Design review of the part built by this model. Coordinates are the model's own, in mm. A direction names the side the tool comes from. Round coordinates to 2 decimals unless told otherwise and drop trailing zeros. Loops run counter-clockwise (first coordinate to the right, second up) from the corner with the lowest first, then second, coordinate; pieces in that order, holes last. Notation, with made-up numbers: (6.25, 88.5) -> (25.25, 88.5) arc R29 ccw to (25.25, 117.5) -> close; hole circle Ø2 at (-39, -1). An arc over 180 degrees is marked (long way). Answer as CSV lines item,"result". Start each with the question number.
(1) Machinability: for faces 4 (the face through (-1.734, 2.262, 145.653)), 5 (the face through (-2.737, 1.61, 72.666)), 6 (the face through (0, -3.175, 73)), 7 (the face through (2.737, -1.61, 72.666)), which of the approach directions +Z, -Z, +X, -X, +Y, -Y give a long, thin tool a straight path to every point of the face, cutting with its end or side? Answer none if there is none.
(2) Take a section at C-C, the plane y = 4.5. Write out the cut boundary in (x, z), and give its area (3 significant figures).
(3) To check wall thickness, follow line 1 (Z direction, x = -6, y = -4); line 2 (Y direction, x = -3.5, z = 48); line 3 (X direction, y = 0.5, z = 144.5). State the ranges of each line that lie inside material, in increasing order. Write a range as from..to.
(4) Draft analysis for pull direction Z (two halves, no side actions). For faces 1 (the face through (0, 0, 159.012)), 2 (the face through (-2.76, -1.57, 72.67)), 3 (the face through (0, 3, 146.312)), state which applies: +Z half, -Z half, draft (parallel to the pull), parting line (faces both ways), or undercut.
(5) Take a section at A-A, the plane x = 0. Write out the cut boundary in (y, z) (3 decimals), and give its area (3 significant figures).
(6) Take a section at B-B, the plane z = 76. Write out the cut boundary in (x, y) (3 decimals).
(7) For P1, Ø4, axis at x = -2.5, z = 112.5, coming from the +Y side (3 decimals); P2, Ø2, axis at x = 1.5, z = 57, coming from the -Y side (3 decimals); P3, Ø6, axis at y = 3.5, z = 107.5, coming from the -X side, all flat-tipped, find the tip position at first contact; note any pin that passes through.
from build123d import *

# Parameters (mm, degrees)
SKETCH1_R          = 9.35
PISTON_DEPTH       = 2.5
ROD_DEPTH          = 159.0119
SKETCH4_R          = 9.35
SKETCH4_R_2        = 3.175
THREAD_DEPTH       = 14
CHAMFER1_SIZE      = 1
SKETCH5_W          = 1.3
SKETCH5_H          = 2.54
CUT_REVOLVE1_ANGLE = 180


with BuildPart() as part:
    # Sketch1 → Piston (new, symmetric)
    with BuildSketch(Plane.XY):
        Circle(SKETCH1_R)
    extrude(amount=PISTON_DEPTH, both=True)

    # Sketch2 → Rod (add)
    with BuildSketch(Plane.XY):
        Polygon((3.666174209, 0), (1.833087105, 3.175), (-1.833087105, 3.175), (-3.666174209, 0), (-1.833087105, -3.175), (1.833087105, -3.175), align=None)
    extrude(amount=ROD_DEPTH)

    # Sketch4 → Thread (cut)
    with BuildSketch(Plane.XY.offset(159.0119)):
        Circle(SKETCH4_R)
        with Locations(Location((0, 0, 0), (0, 0, 330))):
            Circle(SKETCH4_R_2, mode=Mode.SUBTRACT)
    extrude(amount=-THREAD_DEPTH, mode=Mode.SUBTRACT)

    # Chamfer1
    chamfer1_edges = [part.edges().sort_by_distance(p)[0] for p in [
        (-2.749630657, 1.5875, 159.0119),
    ]]
    chamfer(chamfer1_edges, length=CHAMFER1_SIZE)

    # Sketch5 → Cut-Revolve1 (revolve, cut)
    with BuildSketch(Plane(origin=(0, 0, 0), x_dir=(0, 0, -1), z_dir=(1, 0, 0))):
        with Locations((-145.6619, 4.12)):
            Rectangle(SKETCH5_W, SKETCH5_H)
        with Locations((-145.6619, -4.12)):
            Rectangle(SKETCH5_W, SKETCH5_H)
    revolve(axis=Axis((0, 0, 47.288533753), (0, 0, 1)), revolution_arc=CUT_REVOLVE1_ANGLE, mode=Mode.SUBTRACT)

    # Sketch6 → Cut-Revolve2 (revolve, cut)
    with BuildSketch(Plane(origin=(0, 0, 0), x_dir=(0, 0, -1), z_dir=(1, 0, 0)), mode=Mode.PRIVATE) as cut_revolve2_sk:
        Polygon((-145.0119, 2.85), (-145.0119, 7.746831352), (-142.184713101, 7.746831352), align=None)
    revolve(cut_revolve2_sk.sketch.rotate(Axis((0, 0, 96.043182271), (0, 0, 1)), 90), axis=Axis((0, 0, 96.043182271), (0, 0, 1)), mode=Mode.SUBTRACT)


solid = part.part
The answers:
1,face 4,"none"
1,face 5,"+Z, -X, +Y"
1,face 6,"+Z, +X, -X, -Y"
1,face 7,"+Z, +X, -Y"
2,outline,"(-8.2, -2.5) -> (8.2, -2.5) -> (8.2, 2.5) -> (-8.2, 2.5) -> close"
2,area,"82.0 mm²"
3,line 1,"-2.5..2.5"
3,line 2,"-0.29..0.29"
3,line 3,"-3.38..3.38"
4,face 1,"+Z half"
4,face 2,"draft"
4,face 3,"undercut"
5,outline,"(-9.35, -2.5) -> (9.35, -2.5) -> (9.35, 2.5) -> (3.175, 2.5) -> (3.175, 144.824) -> (2.85, 145.012) -> (2.85, 146.312) -> (3.175, 146.312) -> (3.175, 158.012) -> (2.175, 159.012) -> (-2.175, 159.012) -> (-3.175, 158.012) -> (-3.175, 146.312) -> (-2.85, 146.312) -> (-2.85, 145.012) -> (-3.175, 144.824) -> (-3.175, 2.5) -> (-9.35, 2.5) -> close"
5,area,"1,090 mm²"
6,outline,"(-3.666, 0) -> (-1.833, -3.175) -> (1.833, -3.175) -> (3.666, 0) -> (1.833, 3.175) -> (-1.833, 3.175) -> close"
7,P1,"y = 3.175"
7,P2,"y = -3.175"
7,P3,"x = -3.38"
